Design review of the part built by this model. Coordinates are the model's own, in mm. A direction names the side the tool comes from. Coordinates: 2 decimals unless noted, no trailing zeros. Loops run counter-clockwise (first coordinate to the right, second up) from the corner with the lowest first, then second, coordinate; pieces in that order, holes last. Notation, with made-up numbers: M 65.25,73.5 L 91.25,73.5 A16 ccw 91.25,85.5 Z; hole C 84.5,78 d9. An arc over 180 degrees is marked long. Put each result on its own line as item: value. Start each with the question number.
(1) Take a section at C-C, the plane y = 2.5. Count the separate pieces of the cut face and the enclosed holes in it, then the cut area to 3 significant figures.
(2) Take a section at B-B, the plane z = -48. Give the boundary of the cut face in (x, y).
(3) Take a section at A-A, the plane x = -20. Give the boundary of the cut face in (y, z).
(4) For faces 4 (the flat face through (0, 1, -55)), 5 (the flat face through (20, 2, -33.5)), list the 3-axis set-ups (+Z, -Z, +X, -X, +Y, -Y) from which the entire face can be reached by the end or side of a thin tool; tool diameter is ignored.
(5) For probe 1 along X at (y, z) = (1.4, 33); probe 2 along X at (y, z) = (0.3, -2), list the stretches that pass through material, from the lowest coordinate up. Write a range as [from, to].
(6) Clearance check with a flat-ended pin moving along its axis: pin 1 (0.9 mm diameter, centred on y = 2, z = 35.5, fed in from +X). State where the tip first meets the part, or that it passes through.
(7) The part is to be moulded in two halves that separate along X. For faces 1 (the flat face through (-33.5, 2, 0)), 2 (the flat face through (0, 1, 55)), 3 (the cylindrical face through (48.986, 1.521, -49.297)), say which applies: +X half, -X half, draft (parallel to the pull), parting line (faces both ways), or undercut.
```python
from build123d import *

# Parameters (mm, degrees)
SKETCH1_W           = 110
SKETCH1_H           = 110
SKETCH1_R           = 2.5
BOSS_EXTRUDE1_DEPTH = 3
FILLET1_R           = 20
SKETCH2_W           = 3
SKETCH2_H           = 10
SKETCH2_W_2         = 10
SKETCH2_H_2         = 3
CUT_EXTRUDE1_DEPTH  = 78.839578622


with BuildPart() as part:
    # Sketch1 → Boss-Extrude1 (new body)
    with BuildSketch(Plane(origin=(0, 0, 0), x_dir=(1, 0, 0), z_dir=(0, 1, 0))):
        Rectangle(SKETCH1_W, SKETCH1_H)
        with Locations(Location((33, 48, 0), (0, 0, 270))):
            Circle(SKETCH1_R, mode=Mode.SUBTRACT)
        with Locations(Location((-33, 48, 0), (0, 0, 270))):
            Circle(SKETCH1_R, mode=Mode.SUBTRACT)
        with Locations(Location((48, 33, 0), (0, 0, 270))):
            Circle(SKETCH1_R, mode=Mode.SUBTRACT)
        with Locations(Location((48, -33, 0), (0, 0, 270))):
            Circle(SKETCH1_R, mode=Mode.SUBTRACT)
        with Locations(Location((33, -48, 0), (0, 0, 270))):
            Circle(SKETCH1_R, mode=Mode.SUBTRACT)
        with Locations(Location((-33, -48, 0), (0, 0, 270))):
            Circle(SKETCH1_R, mode=Mode.SUBTRACT)
        with Locations(Location((-48, -33, 0), (0, 0, 270))):
            Circle(SKETCH1_R, mode=Mode.SUBTRACT)
        with Locations(Location((-48, 33, 0), (0, 0, 270))):
            Circle(SKETCH1_R, mode=Mode.SUBTRACT)
    extrude(amount=BOSS_EXTRUDE1_DEPTH)

    # Fillet1
    fillet1_edges = [part.edges().sort_by_distance(p)[0] for p in [
        (55, 1.5, 55),
        (-55, 1.5, 55),
        (-55, 1.5, -55),
        (55, 1.5, -55),
    ]]
    fillet(fillet1_edges, radius=FILLET1_R)

    # Sketch2 → Cut-Extrude1 (cut, through all)
    with BuildSketch(Plane(origin=(0, 3, 0), x_dir=(1, 0, 0), z_dir=(0, 1, 0))):
        with Locations((-35, -20)):
            Rectangle(SKETCH2_W, SKETCH2_H)
        with Locations((-35, 0)):
            Rectangle(SKETCH2_W, SKETCH2_H)
        with Locations((-20, 35)):
            Rectangle(SKETCH2_W_2, SKETCH2_H_2)
        with Locations((0, 35)):
            Rectangle(SKETCH2_W_2, SKETCH2_H_2)
        with Locations((20, 35)):
            Rectangle(SKETCH2_W_2, SKETCH2_H_2)
        with Locations((35, 20)):
            Rectangle(SKETCH2_W, SKETCH2_H)
        with Locations((35, 0)):
            Rectangle(SKETCH2_W, SKETCH2_H)
        with Locations((35, -20)):
            Rectangle(SKETCH2_W, SKETCH2_H)
        with Locations((20, -35)):
            Rectangle(SKETCH2_W_2, SKETCH2_H_2)
        with Locations((0, -35)):
            Rectangle(SKETCH2_W_2, SKETCH2_H_2)
        with Locations((-20, -35)):
            Rectangle(SKETCH2_W_2, SKETCH2_H_2)
        with Locations((-35, 20)):
            Rectangle(SKETCH2_W, SKETCH2_H)
    extrude(amount=-CUT_EXTRUDE1_DEPTH, mode=Mode.SUBTRACT)


solid = part.part
```
Computed values:
1. separate pieces: 1
1. enclosed holes: 20
1. area: 11,200 mm^2
2. outline: M -50.2,0 L -35.5,0 L -35.5,3 L -50.2,3 Z; M -30.5,0 L 30.5,0 L 30.5,3 L -30.5,3 Z; M 35.5,0 L 50.2,0 L 50.2,3 L 35.5,3 Z
3. outline: M 0,-55 L 3,-55 L 3,-36.5 L 0,-36.5 Z; M 0,-33.5 L 3,-33.5 L 3,33.5 L 0,33.5 Z; M 0,36.5 L 3,36.5 L 3,55 L 0,55 Z
4. face 4: -Z, +X, -X, +Y, -Y
4. face 5: +Y, -Y
5. probe 1: x = [-55, -50.5], [-45.5, 45.5], [50.5, 55]
5. probe 2: x = [-55, -36.5], [-33.5, 33.5], [36.5, 55]
6. pin 1: stops at x = 55
7. face 1: undercut
7. face 2: draft
7. face 3: +X half
